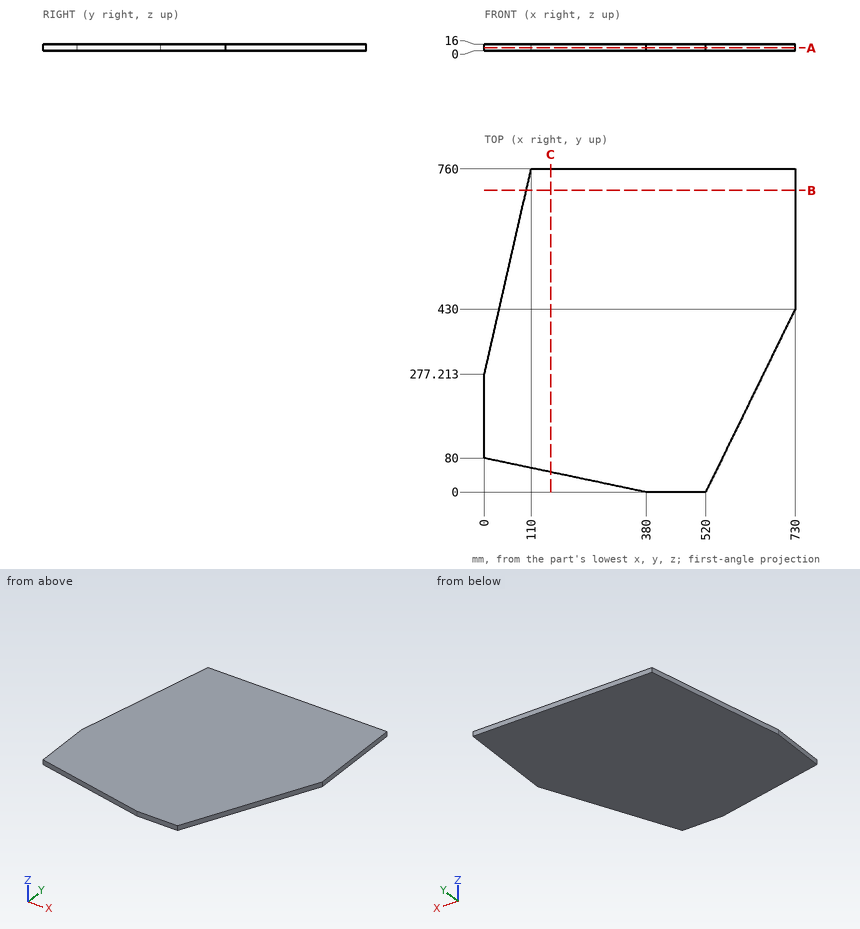
Answer from the drawing. Dimensions are ordinates in mm from the lowest x, y and z of the part. Give positions to 0.01 mm unless a question says otherwise; leave off trailing zeros. Order: outer loops, then holes, each group sorted by start corner. A loop starts at its lowest first (then second) coordinate and runs counter-clockwise, first axis right, second up.
(1) Find section A-A (z = 7). Give the vertices of the cut face in (x, y).
(2) Find section B-B (y = 709.5). Give the vertices of the cut face in (x, z), plus the area to 3 significant figures.
(3) Straight lines are drawn through the part: L1, parallel to X at y = 288.5, z = 6.5 (1 decimal); L2, parallel to Y at x = 631.5, z = 13.5; L3, parallel to X at y = 170.5, z = 7.75. For each, find the intervals that lie inside material, in ascending order.
(4) Given pin 1 (5 mm diameter, centred on x = 420, y = 126, fed in from -Z); pin 2 (1.5 mm diameter, centred on y = 156, z = 11, fed in from +X); pin 3 (6 mm diameter, centred on x = 129.5, z = 9.5, fed in from -Y) (1 decimal); pin 4 (5 mm diameter, centred on y = 538, z = 11, fed in from -X), each flat-ended and moving along its own axis, determine where each tip first touches the part or whether it passes through.
(5) Find section C-C (x = 155.5). Give the vertices of the cut face in (y, z).
Result sheet:
1. outline: (0, 80) - (380, 0) - (520, 0) - (730, 430) - (730, 760) - (110, 760) - (0, 277.21) - close
2. outline: (98.49, 0) - (730, 0) - (730, 16) - (98.49, 16) - close
2. area: 10,100 mm2
3. L1: x = 2.6 to 660.9
3. L2: y = 228.31 to 760
3. L3: x = 0 to 603.27
4. pin 1: stops at z = 0
4. pin 2: stops at x = 596.55
4. pin 3: stops at y = 52.1
4. pin 4: stops at x = 58.85
5. outline: (47.26, 0) - (760, 0) - (760, 16) - (47.26, 16) - close
